from build123d import *

# Parameters (mm, degrees)
F0_W       = 72
F0_H       = 36
F1_DEPTH   = 12
F3_DEPTH   = 50
F5_DEPTH   = 22
F6_W       = 50
F6_H       = 0.5
F7_DEPTH   = 10
F8_DEPTH   = 10
F13_W      = 1
F13_H      = 10
F14_DEPTH  = 1
F15_DEPTH  = 2
F13_W_2    = 34.824172408
F16_DEPTH  = 3
F17_W      = 1
F17_H      = 1
F18_DEPTH  = 8
F19_DEPTH  = 8
F20_DEPTH  = 8
F21_DEPTH  = 8
F22_DEPTH  = 8
F13_H_2    = 1
F23_DEPTH  = 11
F24_DEPTH  = 11
F25_W      = 1
F25_H      = 2.1276606619
F27_DEPTH  = 2
F26_W      = 1
F26_H      = 2.1276606619
F28_DEPTH  = 1
F29_W      = 36
F29_H      = 3.5
F30_DEPTH  = 6
F31_W      = 6
F31_H      = 1
F32_DEPTH  = 2
F33_DEPTH  = 1
F34_DEPTH  = 2
F35_DEPTH  = 1
F37_START  = -4
F37_DEPTH  = 29
F38_W      = 1
F38_H      = 1
F39_DEPTH  = 8.5
F40_DEPTH  = 8.5
F41_DEPTH  = 8.5
F42_DEPTH  = 8.5
F43_DEPTH  = 8.5
F45_W      = 6.2820501626
F45_H      = 5.7211536914
F46_FACE_W = 6.2820501626
F46_FACE_H = 4.3090674287
F47_FACE_W = 6.2820501626
F47_FACE_H = 4.3090674287
F51_W      = 5.2950629033
F51_H      = 9.0086418204


with BuildPart() as f1:
    # F0 (on Top) → F1 (new body)
    with BuildSketch(Plane.XY):
        with Locations((-17.9916281849, -0.2358976454)):
            Rectangle(F0_W, F0_H)
    extrude(amount=F1_DEPTH)

    # F2 (on face) → F3 (join)
    with BuildSketch(Plane.YZ.offset(18.0083718151)):
        Polygon((-18.2358976454, 12), (17.7641023546, 12), (0, 33.9695699513), align=None)
    extrude(amount=-F3_DEPTH)

    # F4 (on face) → F5 (join, through all)
    with BuildSketch(Plane(origin=(-53.9916281849, 0, 0), x_dir=(0, -1, 0), z_dir=(-1, 0, 0))):
        Polygon((0, 19.2015562207), (-17.7641023546, 12), (18.2358976454, 12), align=None)
    extrude(amount=-F5_DEPTH)

    # F6 (on face) → F7 (join)
    with BuildSketch(Plane.XZ.offset(18.2358976454)):
        with Locations((-6.9916281849, 11.75)):
            Rectangle(F6_W, F6_H)
    extrude(amount=F7_DEPTH)

    # F6 (on face) → F8 (join)
    with BuildSketch(Plane.XZ.offset(18.2358976454)):
        with Locations((-6.9916281849, 0.25)):
            Rectangle(F6_W, F6_H)
    extrude(amount=F8_DEPTH)

    # F9 (on face) → F10 (join, up to the next surface of F1)
    with BuildSketch(Plane.XZ.offset(28.2358976454)):
        Polygon((-26.0598938912, 16.733692959), (-31.9916281849, 12), (-20.1281595975, 12), align=None)
    extrude(until=Until.NEXT, dir=(0, 1, 0))

    # F11 (on face) → F12 (join, up to the next surface of F1)
    with BuildSketch(Plane.YZ.offset(18.0083718151)):
        Polygon((-14.3066837157, 16.733692959), (-28.2358976454, 12), (-18.2358976454, 12), align=None)
    extrude(until=Until.NEXT, dir=(-1, 0, 0))

    # F13 (on face) → F14 (join)
    with BuildSketch(Plane.XY.offset(0.5)):
        with Locations((-18.3158005929, -23.2358976454)):
            Rectangle(F13_W, F13_H)
    extrude(amount=F14_DEPTH)

    # F13 (on face) → F15 (join)
    with BuildSketch(Plane.XY.offset(0.5)):
        with Locations((-17.3158005929, -23.2358976454)):
            Rectangle(F13_W, F13_H)
    extrude(amount=F15_DEPTH)

    # F13 (on face) → F16 (join)
    with BuildSketch(Plane.XY.offset(0.5)):
        with Locations((0.5962856111, -23.2358976454)):
            Rectangle(F13_W_2, F13_H)
    extrude(amount=F16_DEPTH)

    # F17 (on face) → F18 (join, through all)
    with BuildSketch(Plane.XY.offset(3.5)):
        with Locations((-14.0816532895, -27.7358976454)):
            Rectangle(F17_W, F17_H)
    extrude(amount=F18_DEPTH)

    # F17 (on face) → F19 (join, through all)
    with BuildSketch(Plane.XY.offset(3.5)):
        with Locations((-8.3204968274, -27.7358976454)):
            Rectangle(F17_W, F17_H)
    extrude(amount=F19_DEPTH)

    # F17 (on face) → F20 (join, through all)
    with BuildSketch(Plane.XY.offset(3.5)):
        with Locations((0.2891260535, -27.7358976454)):
            Rectangle(F17_W, F17_H)
    extrude(amount=F20_DEPTH)

    # F17 (on face) → F21 (join, through all)
    with BuildSketch(Plane.XY.offset(3.5)):
        with Locations((8.8987489343, -27.7358976454)):
            Rectangle(F17_W, F17_H)
    extrude(amount=F21_DEPTH)

    # F17 (on face) → F22 (join, through all)
    with BuildSketch(Plane.XY.offset(3.5)):
        with Locations((17.5083718151, -27.7358976454)):
            Rectangle(F17_W, F17_H)
    extrude(amount=F22_DEPTH)

    # F13 (on face) → F23 (join, through all)
    with BuildSketch(Plane.XY.offset(0.5)):
        with Locations((-31.4916281849, -27.7358976454)):
            Rectangle(F13_W, F13_H_2)
    extrude(amount=F23_DEPTH)

    # F13 (on face) → F24 (join, through all)
    with BuildSketch(Plane.XY.offset(0.5)):
        with Locations((-23.9017895311, -27.7358976454)):
            Rectangle(F13_W, F13_H_2)
    extrude(amount=F24_DEPTH)

    # F25 (on face) → F27 (join)
    with BuildSketch(Plane.XY.offset(1.5)):
        with Locations((-18.3158005929, -27.1720673144)):
            Rectangle(F25_W, F25_H)
    extrude(amount=F27_DEPTH)

    # F26 (on face) → F28 (join)
    with BuildSketch(Plane.XY.offset(2.5)):
        with Locations((-17.3158005929, -27.1720673144)):
            Rectangle(F26_W, F26_H)
    extrude(amount=F28_DEPTH)

    # F29 (on face) → F30 (join)
    with BuildSketch(Plane.YZ.offset(18.0083718151)):
        with Locations((-0.2358976454, 1.75)):
            Rectangle(F29_W, F29_H)
    extrude(amount=F30_DEPTH)

    # F31 (on face) → F32 (cut)
    with BuildSketch(Plane.XY.offset(3.5)):
        with Locations((21.0083718151, -17.7358976454)):
            Rectangle(F31_W, F31_H)
    extrude(amount=-F32_DEPTH, mode=Mode.SUBTRACT)

    # F31 (on face) → F33 (cut)
    with BuildSketch(Plane.XY.offset(3.5)):
        with Locations((21.0083718151, -16.7358976454)):
            Rectangle(F31_W, F31_H)
    extrude(amount=-F33_DEPTH, mode=Mode.SUBTRACT)

    # F31 (on face) → F34 (cut)
    with BuildSketch(Plane.XY.offset(3.5)):
        with Locations((21.0083718151, 17.2641023546)):
            Rectangle(F31_W, F31_H)
    extrude(amount=-F34_DEPTH, mode=Mode.SUBTRACT)

    # F31 (on face) → F35 (cut)
    with BuildSketch(Plane.XY.offset(3.5)):
        with Locations((21.0083718151, 16.2641023546)):
            Rectangle(F31_W, F31_H)
    extrude(amount=-F35_DEPTH, mode=Mode.SUBTRACT)

    # F36 (on face) → F37 (join)
    with BuildSketch(Plane(origin=(0, 17.7641023546, 0), x_dir=(-1, 0, 0), z_dir=(0, 1, 0)).offset(F37_START)):
        Polygon((-18.0083718151, 12), (-18.0083718151, 16.4085291326), (-24.0083718151, 12), align=None)
    extrude(amount=-F37_DEPTH)

    # F38 (on face) → F39 (join, through all)
    with BuildSketch(Plane.XY.offset(3.5)):
        with Locations((23.5083718151, -14.7358976454)):
            Rectangle(F38_W, F38_H)
    extrude(amount=F39_DEPTH)

    # F38 (on face) → F40 (join, through all)
    with BuildSketch(Plane.XY.offset(3.5)):
        with Locations((23.5083718151, -7.7358976454)):
            Rectangle(F38_W, F38_H)
    extrude(amount=F40_DEPTH)

    # F38 (on face) → F41 (join, through all)
    with BuildSketch(Plane.XY.offset(3.5)):
        with Locations((23.5083718151, -0.7358976454)):
            Rectangle(F38_W, F38_H)
    extrude(amount=F41_DEPTH)

    # F38 (on face) → F42 (join, through all)
    with BuildSketch(Plane.XY.offset(3.5)):
        with Locations((23.5083718151, 6.2641023546)):
            Rectangle(F38_W, F38_H)
    extrude(amount=F42_DEPTH)

    # F38 (on face) → F43 (join, through all)
    with BuildSketch(Plane.XY.offset(3.5)):
        with Locations((23.5083718151, 13.2641023546)):
            Rectangle(F38_W, F38_H)
    extrude(amount=F43_DEPTH)

    # F45 (on offset) → F46 (join, up to the next surface of F1)
    with BuildSketch(Plane.XZ.offset(15)):
        with Locations((-18.8506031036, 23.9503206685)):
            Rectangle(F45_W, F45_H)
        Polygon((-18.8506031036, 30.4006431252), (-21.9916281849, 26.8108975142), (-15.7095780224, 26.8108975142), align=None)
    extrude(until=Until.NEXT, dir=(0, 1, 0))

    # F45 (on offset) → F47 (join, up to the next surface of F1)
    with BuildSketch(Plane.XZ.offset(15)):
        with Locations((4.8673467338, 23.9503206685)):
            Rectangle(F45_W, F45_H)
        Polygon((4.8673467338, 30.4006431252), (1.7263216525, 26.8108975142), (8.0083718151, 26.8108975142), align=None)
    extrude(until=Until.NEXT, dir=(0, 1, 0))

    # F46_face (on face) → F48 (join, up to the next surface of F1)
    with BuildSketch(Plane(origin=(-18.8506031036, -12.8454662856, 21.0897438228), x_dir=(1, 0, 0), z_dir=(0, 0, -1))):
        Rectangle(F46_FACE_W, F46_FACE_H)
    extrude(until=Until.NEXT)

    # F47_face (on face) → F49 (join, up to the next surface of F1)
    with BuildSketch(Plane(origin=(4.8673467338, -12.8454662856, 21.0897438228), x_dir=(1, 0, 0), z_dir=(0, 0, -1))):
        Rectangle(F47_FACE_W, F47_FACE_H)
    extrude(until=Until.NEXT)

    # F51 (on offset) → F52 (join, up to the next surface of F1)
    with BuildSketch(Plane.XY.offset(40)):
        with Locations((-2.6475314517, -8.4023226518)):
            Rectangle(F51_W, F51_H)
    extrude(until=Until.NEXT, dir=(0, 0, -1))


solid = f1.part
For this review, take the finished solid that the model builds, in its own axes (mm). A direction names the side the tool comes from. Round coordinates to 2 decimals unless told otherwise and drop trailing zeros. Order: outer loops, then holes, each group sorted by start corner. A loop starts at its lowest first (then second) coordinate and runs counter-clockwise, first axis right, second up. Notation, with made-up numbers: (-38.75, 19.25) -> (-0.75, 19.25) arc R32 ccw to (-0.75, 57.25) -> close; hole circle Ø8 at (-14.5, 62.25). An arc over 180 degrees is marked (long way). Write item = value, one per line. Start each with the question number.
1) To check wall thickness, follow line 1 (X direction, y = -13.5, z = 18); line 2 (Y direction, x = 0, z = 5); line 3 (X direction, y = -7.5, z = 9). State the ranges of each line that lie inside material, in increasing order. Write a range as from..to.
2) The part is to be moulded in two halves that separate along X. For faces 1 (the face through (-16, -6, 0)), 2 (the face through (-31.992, 0, 21)), 3 (the face through (3.32, -10.4, 28.63)), say which applies: +X half, -X half, draft (parallel to the pull), parting line (faces both ways), or undercut.
3) Take a section at A-A on y = -25. State the section outline as (x, z) points.
4) Take a section at B-B on z = 32. State the section outline as (x, y) points.
5) Tool access review of faces 4 (the face through (-18.816, -24, 1)), 5 (the face through (-43.15, 8.76, 15.65)), 6 (the face through (1.726, -11, 23)), 7 (the face through (21.9, -15.236, 12.3)), 8 (the face through (-31.992, -28, 6)): name each direction out of +Z, -Z, +X, -X, +Y, -Y from which nothing blocks a thin tool from reaching the whole face with its end or side.
6) Take a section at C-C on x = 16. State the section outline as (y, z) points.
7) Take a section at D-D on z = 6.5. Count the separate pieces of the cut face and the enclosed holes in it, plus the area to 3 significant figures.
8) Insertion check: pin 1 (1.1 mm diameter, centred on y = -28, z = 6.5, fed in from -X); pin 2 (0.5 mm diameter, centred on x = -17.5, y = -20.5, fed in from +Z); pin 3 (1.1 mm diameter, centred on y = -28, z = 4, fed in from +X). Each pin has a flat end and moves straight along its axis. Give the tip position at first contact, or say it passes through.
Verdict:
q1.line_1 = -21.99..-15.71, 1.73..8.01
q1.line_2 = -28.24..-27.24, -18.24..17.76
q1.line_3 = -53.99..18.01, 23.01..24.01
q2.face_1 = draft
q2.face_2 = -X half
q2.face_3 = undercut
q3.outline = (-31.99, 0) -> (18.01, 0) -> (18.01, 3.5) -> (-16.82, 3.5) -> (-16.82, 2.5) -> (-17.82, 2.5) -> (-17.82, 1.5) -> (-18.82, 1.5) -> (-18.82, 0.5) -> (-31.99, 0.5) -> close; (-31.99, 11.5) -> (18.01, 11.5) -> (18.01, 13.1) -> (-21.51, 13.1) -> (-26.06, 16.73) -> (-31.99, 12) -> close
q4.outline = (-31.99, -1.63) -> (18.01, -1.63) -> (18.01, 1.59) -> (-31.99, 1.59) -> close; (-5.3, -12.91) -> (0, -12.91) -> (0, -3.9) -> (-5.3, -3.9) -> close
q5.face_4 = -Y
q5.face_5 = +Z, -X, +Y
q5.face_6 = +Z, -Y
q5.face_7 = +Z, +X, -Y
q5.face_8 = +Z, -Z, -X, -Y
q6.outline = (-28.24, 0) -> (17.76, 0) -> (17.76, 12) -> (0, 33.97) -> (-14.31, 16.73) -> (-28.24, 12) -> (-28.24, 11.5) -> (-18.24, 11.5) -> (-18.24, 3.5) -> (-28.24, 3.5) -> close
q7.separate_pieces = 13
q7.enclosed_holes = 0
q7.area = 2,600 mm2
q8.pin_1 = -31.99
q8.pin_2 = 14.71
q8.pin_3 = 18.01
